Design review of the part built by this model. Coordinates are the model's own, in mm. Face numbers are marked on the shaded views. A direction names the side the tool comes from. Give positions to 0.01 mm unless a question says otherwise; leave off trailing zeros. Write each loop counter-clockwise with the first axis right and the second up, starting at its lowest first coordinate (ties: lowest second). Pieces come first, ordered by that corner, then holes. Notation, with made-up numbers: M 68,-17.5 L 85,-17.5 A36 ccw 85,20.5 Z; hole C -23,26 d6. An arc over 180 degrees is marked long. Answer in a Markdown table with one row per item.
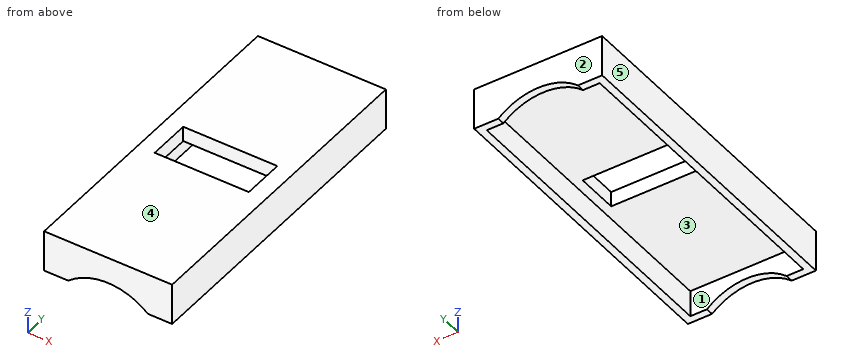
```python
from build123d import *

# Parameters (mm, degrees)
CYLINDER004_R     = 8
CYLINDER004_DEPTH = 45
BOX007_W          = 15
BOX007_H          = 40
BOX007_DEPTH      = 5.5
BOX006_W          = 17
BOX006_H          = 42
BOX006_DEPTH      = 5.5
BOX002_W          = 12.5
BOX002_H          = 5.6
BOX002_DEPTH      = 10
BOX005_W          = 15
BOX005_H          = 40
BOX005_DEPTH      = 2


with BuildPart() as cylinder004:
    # Cylinder004 → Cylinder004 (new body)
    with BuildSketch(Plane(origin=(6, -19.5, -6), x_dir=(1, 0, 0), z_dir=(0, 1, 0))):
        Circle(CYLINDER004_R)
    extrude(amount=CYLINDER004_DEPTH)


with BuildPart() as cube007:
    # Box007 → Box007 (new body)
    with BuildSketch(Plane(origin=(-1.5, -17.3, 0), x_dir=(1, 0, 0), z_dir=(0, 0, 1))):
        with Locations((7.5, 20)):
            Rectangle(BOX007_W, BOX007_H)
    extrude(amount=BOX007_DEPTH)


with BuildPart() as cut008:
    # Box006 → Box006 (new body)
    with BuildSketch(Plane(origin=(-2.5, -18.3, 0), x_dir=(1, 0, 0), z_dir=(0, 0, 1))):
        with Locations((8.5, 21)):
            Rectangle(BOX006_W, BOX006_H)
    extrude(amount=BOX006_DEPTH)

    # Cut008: cut Cube007
    add(cube007.part, mode=Mode.SUBTRACT)


with BuildPart() as cube002:
    # Box002 → Box002 (new body)
    with BuildSketch(Plane(origin=(-0.25, 0.1, 0), x_dir=(1, 0, 0), z_dir=(0, 0, 1))):
        with Locations((6.25, 2.8)):
            Rectangle(BOX002_W, BOX002_H)
    extrude(amount=BOX002_DEPTH)


with BuildPart() as obj1:
    # Box005 → Box005 (new body)
    with BuildSketch(Plane(origin=(-1.5, -17.3, 0), x_dir=(1, 0, 0), z_dir=(0, 0, 1))):
        with Locations((7.5, 20)):
            Rectangle(BOX005_W, BOX005_H)
    extrude(amount=BOX005_DEPTH)

    # Cut007: cut Cube002
    add(cube002.part, mode=Mode.SUBTRACT)


with BuildPart() as obj1_1:
    # Cut007 placement: moved
    add(obj1.part.moved(Location((0, 0, 3.5))))

    # Fusion003: union Cut008
    add(cut008.part)

    # Cut015: cut Cylinder004
    add(cylinder004.part, mode=Mode.SUBTRACT)


solid = obj1_1.part
```
1) Add section C-C (y = 20). Write out the cut boundary in (x, z), and give its area (3 significant figures).
Geometry says:
| item | result |
|---|---|
| outline | M -2.5,0 L -1.5,0 L -1.5,3.5 L 13.5,3.5 L 13.5,0 L 14.5,0 L 14.5,5.5 L -2.5,5.5 Z |
| area | 41.0 mm^2 |
2) The part is to be moulded in two halves that separate along Z. For the marked faces 3, 4 and 5, say which applies: released by +Z, released by -Z, zero draft, split by the parting line, or undercut.
Geometry says:
| item | result |
|---|---|
| face 3 | released by -Z |
| face 4 | released by +Z |
| face 5 | zero draft |
3) Add section A-A (x = 2.25). Write out the cut boundary in (y, z).
Geometry says:
| item | result |
|---|---|
| outline | M -18.3,1.07 L -17.3,1.07 L -17.3,3.5 L 0.1,3.5 L 0.1,5.5 L -18.3,5.5 Z; M 5.7,3.5 L 22.7,3.5 L 22.7,1.07 L 23.7,1.07 L 23.7,5.5 L 5.7,5.5 Z |
4) To check wall thickness, follow probe 1 along X at (y, z) = (14.5, 0.45); probe 2 along Y at (x, z) = (1.75, 4.1); probe 3 along Y at (x, z) = (3, 3.35). State the ranges of each line that lie inside material, in increasing order. Write a range as [from, to].
Geometry says:
| item | result |
|---|---|
| probe 1 | [-2.5, -1.5], [13.5, 14.5] |
| probe 2 | [-18.3, 0.1], [5.7, 23.7] |
| probe 3 | [-18.3, -17.3], [22.7, 23.7] |
5) Add section B-B (z = 1.2). Write out the cut boundary in (x, y).
Geometry says:
| item | result |
|---|---|
| outline | M -2.5,-18.3 L 2.51,-18.3 L 2.51,-17.3 L -1.5,-17.3 L -1.5,22.7 L 2.51,22.7 L 2.51,23.7 L -2.5,23.7 Z; M 9.49,-18.3 L 14.5,-18.3 L 14.5,23.7 L 9.49,23.7 L 9.49,22.7 L 13.5,22.7 L 13.5,-17.3 L 9.49,-17.3 Z |
6) Add section D-D (x = 9.5). Write out the cut boundary in (y, z).
Geometry says:
| item | result |
|---|---|
| outline | M -18.3,1.19 L -17.3,1.19 L -17.3,3.5 L 0.1,3.5 L 0.1,5.5 L -18.3,5.5 Z; M 5.7,3.5 L 22.7,3.5 L 22.7,1.19 L 23.7,1.19 L 23.7,5.5 L 5.7,5.5 Z |
7) For the marked faces 1 and 2, list the 3-axis set-ups (+Z, -Z, +X, -X, +Y, -Y) from which the entire face can be reached by the end or side of a thin tool; tool diameter is ignored.
Geometry says:
| item | result |
|---|---|
| face 1 | -Z |
| face 2 | +Z, -Z, +X, -X, +Y |
